Can you work these out from the drawing? Everything is in mm from the part's minimum corner. Coordinates: 2 decimals unless noted, no trailing zeros. Write each loop counter-clockwise with the first axis right and the second up, starting at its lowest first coordinate (ties: lowest second). Pieces come first, ordered by that corner, then holes.
(1) Please list where these lines run through material, in increasing order: probe 1 along Y at (x, z) = (41, 0.95); probe 2 along Y at (x, z) = (7, 2.9); probe 3 along X at (y, z) = (50, 2.65).
(2) For pin 1 Ø2.5 at (x, z) = (105, 1.5) entering from -Y; pin 2 Ø1.5 at (x, z) = (37, 3.5) entering from +Y; pin 3 Ø2.5 at (y, z) = (3.5, 2) entering from -X, each with a flat end and sliding along its axis, tell me the tip position at first contact or that it passes through.
(3) Imagine slicing it at C-C, the plane y = 55.5. List the corners of the cut face in (x, z) for me.
(4) Imagine slicing it at B-B, the plane x = 34.5. List the corners of the cut face in (y, z) for me, plus the area to 3 significant figures.
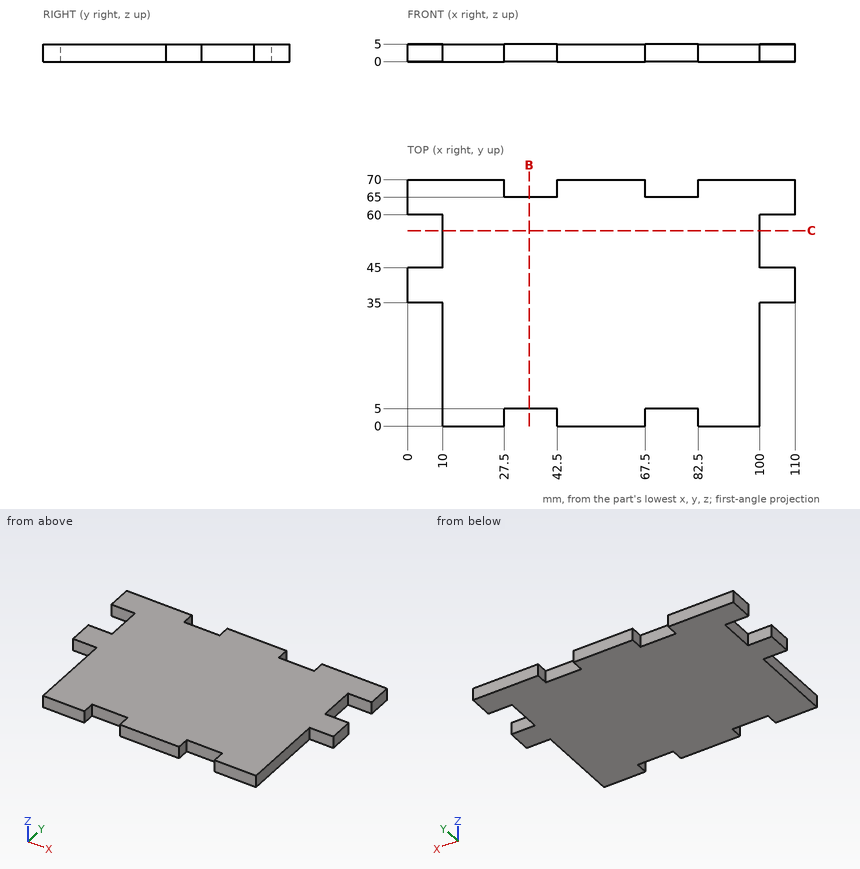
Recorded:
1. probe 1: y = 5 to 65
1. probe 2: y = 35 to 45, 60 to 70
1. probe 3: x = 10 to 100
2. pin 1: stops at y = 35
2. pin 2: stops at y = 65
2. pin 3: stops at x = 10
3. outline: (10, 0) - (100, 0) - (100, 5) - (10, 5) - close
4. outline: (5, 0) - (65, 0) - (65, 5) - (5, 5) - close
4. area: 300 mm2
